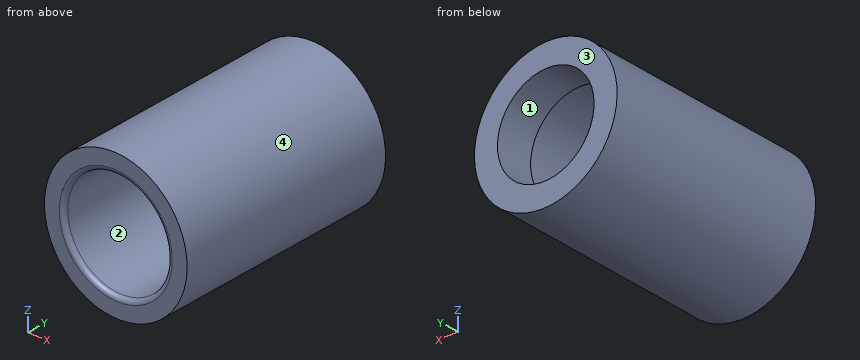
```python
from build123d import *

# Parameters (mm, degrees)
CROQUIS1_R              = 4.8
CROQUIS1_R_2            = 3.5
SALIENTE_EXTRUIR1_DEPTH = 15
CROQUIS2_R              = 3.866185222
CROQUIS2_R_2            = 3.25
SALIENTE_EXTRUIR2_DEPTH = 2.5
REDONDEO1_R             = 0.3


with BuildPart() as part:
    # Croquis1 → Saliente-Extruir1 (new body)
    with BuildSketch(Plane(origin=(0, 0, 0), x_dir=(1, 0, 0), z_dir=(0, 1, 0))):
        with Locations(Location((0, 0, 0), (0, 0, 270))):
            Circle(CROQUIS1_R)
        with Locations(Location((0, 0, 0), (0, 0, 270))):
            Circle(CROQUIS1_R_2, mode=Mode.SUBTRACT)
    extrude(amount=SALIENTE_EXTRUIR1_DEPTH)

    # Croquis2 → Saliente-Extruir2 (add)
    with BuildSketch(Plane(origin=(0, 15, 0), x_dir=(1, 0, 0), z_dir=(0, 1, 0))):
        Circle(CROQUIS2_R)
        with Locations(Location((0, 0, 0), (0, 0, 270))):
            Circle(CROQUIS2_R_2, mode=Mode.SUBTRACT)
    extrude(amount=-SALIENTE_EXTRUIR2_DEPTH)

    # Redondeo1
    redondeo1_edges = [part.edges().sort_by_distance(p)[0] for p in [
        (0, 0, -3.5),
    ]]
    fillet(redondeo1_edges, radius=REDONDEO1_R)


solid = part.part
```
Geometry check sheet. Reference: the model listing, model coordinates, mm. Face numbers are marked on the shaded views. Coordinates: 2 decimals unless noted, no trailing zeros. Write each loop counter-clockwise with the first axis right and the second up, starting at its lowest first coordinate (ties: lowest second). Pieces come first, ordered by that corner, then holes. Notation, with made-up numbers: M 83,68.25 L 106,68.25 A12 cw 106,86.25 Z; hole C -23.5,49 d2. An arc over 180 degrees is marked long. Use one line per item in the form item = value. Start each with the question number.
1) Release check for a two-part mould opening along Z. For the marked faces 1, 2, 3 and 4 record: pulls with the +Z half, pulls with the -Z half, needs draft (parallel to the pull), parting line crosses it, or undercut.
2) Section check C-C on y = 10. Enter the section's corners in (x, z), and give its area (3 significant figures).
3) Section check B-B on x = 0. Enter the section's corners in (y, z), and give its area (3 significant figures).
4) Thickness scan on probe 1 along X at (y, z) = (7.25, 0); probe 2 along X at (y, z) = (13.95, 0); probe 3 along Y at (x, z) = (-3, -1.5). Record the ranges inside material, lowest first. Write a range as from..to.
5) Section check A-A on z = 0. Enter the section's corners in (x, y).
6) Go/stop test with flat-tipped pins: pin 1 Ø1.5 at (x, y) = (-3.5, 12.5) entering from +Z; pin 2 Ø2 at (y, z) = (2, -2) entering from +X; pin 3 Ø4 at (y, z) = (2.5, -3.5) entering from -X. Record where each tip stops, or that it passes through.
Responses:
q1.face_1 = undercut
q1.face_2 = undercut
q1.face_3 = needs draft
q1.face_4 = parting line crosses it
q2.outline = C 0,0 d9.6; hole C 0,0 d7
q2.area = 33.9 mm2
q3.outline = M 0,-4.8 L 15,-4.8 L 15,-3.25 L 12.5,-3.25 L 12.5,-3.5 L 0.3,-3.5 A0.3 ccw 0,-3.8 Z; M 0,3.8 A0.3 ccw 0.3,3.5 L 12.5,3.5 L 12.5,3.25 L 15,3.25 L 15,4.8 L 0,4.8 Z
q3.area = 40.2 mm2
q4.probe_1 = -4.8..-3.5, 3.5..4.8
q4.probe_2 = -4.8..-3.25, 3.25..4.8
q4.probe_3 = 12.5..15
q5.outline = M -4.8,0 L -3.8,0 A0.3 ccw -3.5,0.3 L -3.5,12.5 L -3.25,12.5 L -3.25,15 L -4.8,15 Z; M 3.25,12.5 L 3.5,12.5 L 3.5,0.3 A0.3 ccw 3.8,0 L 4.8,0 L 4.8,15 L 3.25,15 Z
q6.pin_1 = 3.93
q6.pin_2 = 4.69
q6.pin_3 = -4.56
